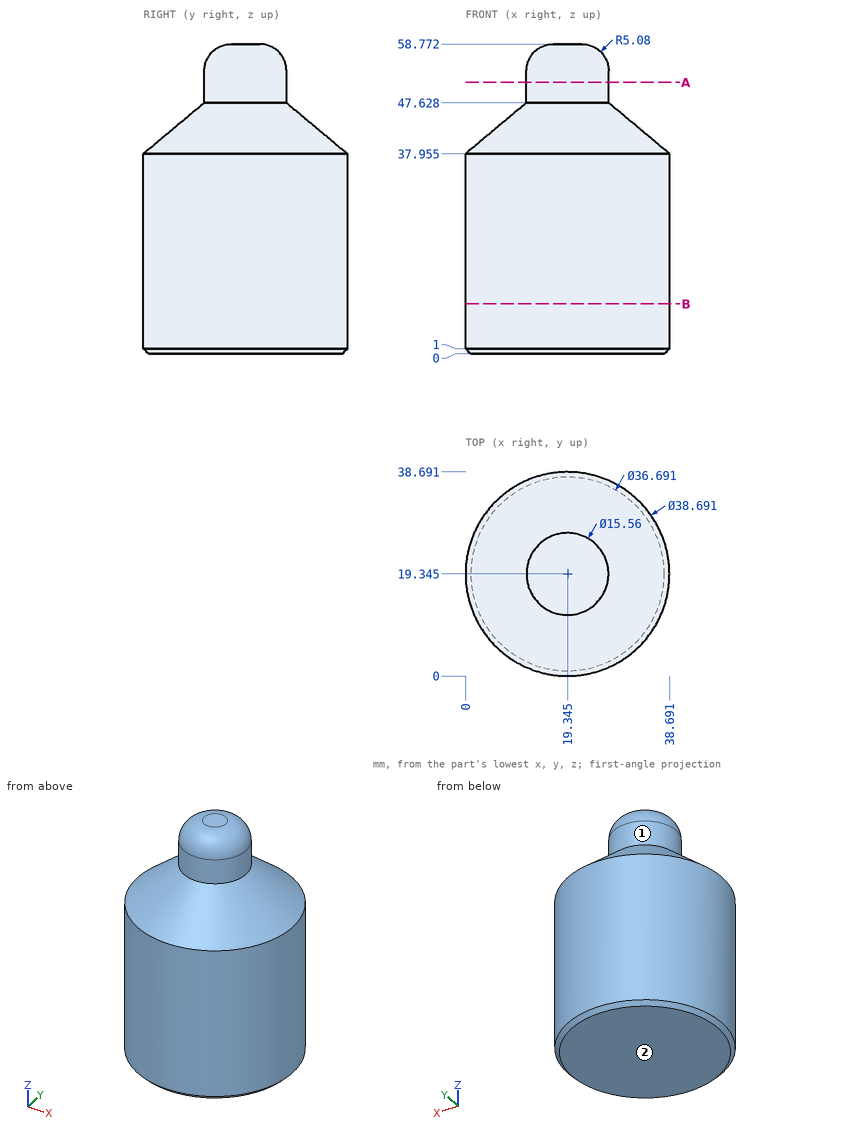
Job drawing, mm, ordinate dimensions from the low corner. One solid piece. A direction names the side the tool comes from. Give positions to 0.01 mm unless a question says otherwise; leave off trailing zeros. Loops run counter-clockwise (first coordinate to the right, second up) from the corner with the lowest first, then second, coordinate; pieces in that order, holes last. Notation, with made-up numbers: M -19.75,-8 L -13.75,-8 A22 cw -13.75,0 Z; hole C 83.25,-34.5 d6. An arc over 180 degrees is marked long. Return JSON: item names as keys, results as strings.
1) Drill centre lines: line 1 (Y direction, x = 19.5, z = 37.5); line 2 (Y direction, x = 19, z = 49.5); line 3 (X direction, y = 22, z = 23.5). Where is each one in solid material? Low to high.
Calculated:
{"line 1": "y = 0 to 38.69", "line 2": "y = 11.57 to 27.12", "line 3": "x = 0.18 to 38.51"}
2) Flat gauge pins, fed straight in: pin 1 Ø8 at (y, z) = (27, 49.5) entering from -X; pin 2 Ø5 at (x, z) = (5, 29) entering from -Y; pin 3 Ø3 at (x, z) = (9.5, 11) entering from +Y. Where does each tip first touch, or does it go through?
Calculated:
{"pin 1": "stops at x = 11.47", "pin 2": "stops at y = 4.05", "pin 3": "stops at y = 36.8"}
3) 3-axis set-ups, long thin cutter, end or side, ignore diameter. For the marked faces 1 and 2: which of +Z, -Z, +X, -X, +Y, -Y reach the whole face in a straight line?
Calculated:
{"face 1": "+Z", "face 2": "-Z, +X, -X, +Y, -Y"}
4) Saw through at B-B, the plane z = 9.5. List the corners of the cut face in (x, y) (1 decimal), then the cut area to 3 significant figures.
Calculated:
{"outline": "C 19.3,19.3 d38.7", "area": "1,180 mm2"}
5) Saw through at A-A, the plane z = 51.5. List the corners of the cut face in (x, y) (1 decimal), then the cut area to 3 significant figures.
Calculated:
{"outline": "C 19.3,19.3 d15.6", "area": "190 mm2"}
